Build history of the part. All positions in model axes, mm. Give positions to 0.01 mm unless a question says otherwise; leave off trailing zeros. Order: outer loops, then holes, each group sorted by start corner. A loop starts at its lowest first (then second) coordinate and runs counter-clockwise, first axis right, second up. Notation, with made-up numbers: M -9,-6 L 26,-6 A25 ccw 26,13 Z; hole C -1,-9 d3. An arc over 180 degrees is marked long. One line per item, written item: value.
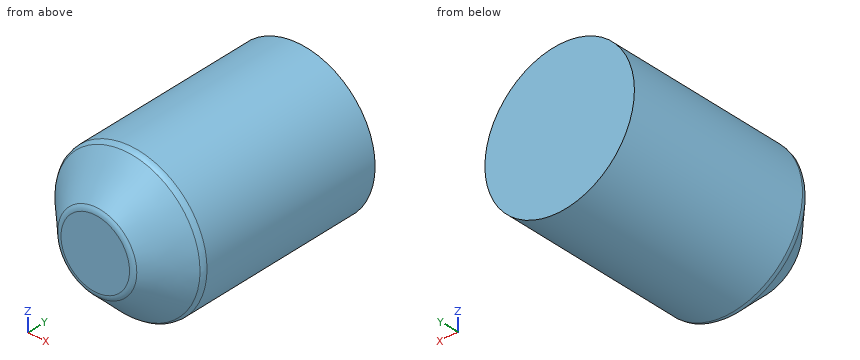
from build123d import *

# Parameters (mm, degrees)
F0_R     = 50
F1_DEPTH = 150
F2_SIZE  = 25
F3_R     = 5


with BuildPart() as f1:
    # F0 (on Front) → F1 (new body)
    with BuildSketch(Plane.XZ):
        Circle(F0_R)
    extrude(amount=F1_DEPTH)

    # F2
    f2_edges = [f1.edges().sort_by_distance(p)[0] for p in [
        (-50, -150, 0),
    ]]
    chamfer(f2_edges, length=F2_SIZE)

    # F3
    f3_edges = [f1.edges().sort_by_distance(p)[0] for p in [
        (37.5, -137.5, 0),
        (-50, -125, 0),
        (-25, -150, 0),
    ]]
    fillet(f3_edges, radius=F3_R)


solid = f1.part
1) Saw through at B-B, the plane y = -131. Write the cut outline in (x, z).
Check values:
outline: C 0,0 d88
2) Pin check, flat tips, straight feed: pin 1 (1.5 mm diameter, centred on x = 2.5, y = -49, fed in from -Z); pin 2 (12 mm diameter, centred on x = 9, y = -118, fed in from +Z); pin 3 (8 mm diameter, centred on y = -47.5, z = -20, fed in from +X). Stop position of each tip, or through.
Check values:
pin 1: z = -49.97
pin 2: z = 49.91
pin 3: x = 47.37
3) Saw through at A-A, the plane y = -29. Write the cut outline in (x, z), then the cut area to 3 significant figures.
Check values:
outline: C 0,0 d100
area: 7,850 mm^2
4) Drill centre lines: probe 1 along Z at (x, y) = (-21, -54); probe 2 along X at (y, z) = (-31, -25.5); probe 3 along Z at (x, y) = (-12, -137). Where is each one in solid material? Low to high. Write a range as from..to.
Check values:
probe 1: -45.38..45.38
probe 2: -43.01..43.01
probe 3: -36.06..36.06
